Could you check a few things on this model? Use its own coordinates, in mm. A direction names the side the tool comes from. Give positions to 0.01 mm unless a question says otherwise; leave off trailing zeros. Order: outer loops, then holes, each group sorted by start corner. A loop starts at its lowest first (then second) coordinate and runs counter-clockwise, first axis right, second up.
from build123d import *

# Parameters (mm, degrees)
F1_DEPTH = 5
F3_DEPTH = 3
F4_DEPTH = 16


with BuildPart() as f1:
    # F0 (on Front) → F1 (new body, symmetric)
    with BuildSketch(Plane.XZ):
        with BuildLine():
            ThreePointArc((0, -4), (-4, 0), (0, 4))
            Line((0, 4), (0, 8))
            ThreePointArc((0, 8), (-6.9282032303, 4), (-6.9282032303, -4))
            Line((-6.9282032303, -4), (0, -4))
        make_face()
        with BuildLine():
            Line((31.6095426679, 8), (0, 8))
            ThreePointArc((0, 8), (4, 6.9282032303), (6.9282032303, 4))
            Line((6.9282032303, 4), (31.6095426679, 4))
            Line((31.6095426679, 4), (31.6095426679, 8))
        make_face()
        with BuildLine():
            Line((0, 8), (0, 4))
            Line((0, 4), (2.413712136, 4))
            Line((2.413712136, 4), (6.9282032303, 4))
            ThreePointArc((6.9282032303, 4), (4, 6.9282032303), (0, 8))
        make_face()
        with BuildLine():
            Line((31.6095426679, -4), (6.9282032303, -4))
            ThreePointArc((6.9282032303, -4), (4.4598401279, -6.6415228701), (1.0806620306, -7.9266745597))
            Line((1.0806620306, -7.9266745597), (31.6095426679, -7.9266745597))
            Line((31.6095426679, -7.9266745597), (31.6095426679, -4))
        make_face()
        with BuildLine():
            ThreePointArc((-1.0806620306, -7.9266745597), (-4.4598401279, -6.6415228701), (-6.9282032303, -4))
            Line((-6.9282032303, -4), (-40.4233634472, -4))
            Line((-40.4233634472, -4), (-40.4233634472, -7.9266745597))
            Line((-40.4233634472, -7.9266745597), (-1.0806620306, -7.9266745597))
        make_face()
        with BuildLine():
            Line((0, -7.9266745597), (0, -4))
            Line((0, -4), (-6.9282032303, -4))
            ThreePointArc((-6.9282032303, -4), (-4.4598401279, -6.6415228701), (-1.0806620306, -7.9266745597))
            Line((-1.0806620306, -7.9266745597), (0, -7.9266745597))
        make_face()
        with BuildLine():
            Line((2.413712136, -4), (0, -4))
            Line((0, -4), (0, -7.9266745597))
            Line((0, -7.9266745597), (1.0806620306, -7.9266745597))
            ThreePointArc((1.0806620306, -7.9266745597), (4.4598401279, -6.6415228701), (6.9282032303, -4))
            Line((6.9282032303, -4), (2.413712136, -4))
        make_face()
        with BuildLine():
            Line((2.413712136, 4), (2.413712136, 3.1896698457))
            Line((2.413712136, 3.1896698457), (7.3366209031, 3.1896698457))
            ThreePointArc((7.3366209031, 3.1896698457), (7.1439107377, 3.6006304131), (6.9282032303, 4))
            Line((6.9282032303, 4), (2.413712136, 4))
        make_face()
        with BuildLine():
            ThreePointArc((6.9282032303, 4), (7.1439107377, 3.6006304131), (7.3366209031, 3.1896698457))
            Line((7.3366209031, 3.1896698457), (31.6095426679, 3.1896698457))
            Line((31.6095426679, 3.1896698457), (31.6095426679, 4))
            Line((31.6095426679, 4), (6.9282032303, 4))
        make_face()
        with BuildLine():
            Line((7.3366209031, -3.1896698457), (2.413712136, -3.1896698457))
            Line((2.413712136, -3.1896698457), (2.413712136, -4))
            Line((2.413712136, -4), (6.9282032303, -4))
            ThreePointArc((6.9282032303, -4), (7.1439107377, -3.6006304131), (7.3366209031, -3.1896698457))
        make_face()
        with BuildLine():
            Line((2.413712136, -4), (2.413712136, -3.1896698457))
            ThreePointArc((2.413712136, -3.1896698457), (1.2730515734, -3.7920099804), (0, -4))
            Line((0, -4), (2.413712136, -4))
        make_face()
        with BuildLine():
            ThreePointArc((0, 4), (1.2730515734, 3.7920099804), (2.413712136, 3.1896698457))
            Line((2.413712136, 3.1896698457), (2.413712136, 4))
            Line((2.413712136, 4), (0, 4))
        make_face()
        with BuildLine():
            Line((31.6095426679, -3.1896698457), (7.3366209031, -3.1896698457))
            ThreePointArc((7.3366209031, -3.1896698457), (7.1439107377, -3.6006304131), (6.9282032303, -4))
            Line((6.9282032303, -4), (31.6095426679, -4))
            Line((31.6095426679, -4), (31.6095426679, -3.1896698457))
        make_face()
    extrude(amount=F1_DEPTH, both=True)

    # F2 (on face) → F3 (join)
    with BuildSketch(Plane.XY.offset(8)):
        Polygon((26.3679362833, -2.1467979489), (26.3679362833, 2.1467979489), (22.6495731622, 4.2935958979), (18.931210041, 2.1467979489), (18.931210041, -2.1467979489), (22.6495731622, -4.2935958979), align=None)
        Polygon((23.6495732055, 1.7320507826), (24.6495731622, 1.1547005384), (24.6495731622, 0), (24.6495731622, -1.1547005384), (23.6495731174, -1.7320508334), (22.6495731622, -2.3094010768), (21.6495731189, -1.7320507826), (20.6495731622, -1.1547005384), (20.6495731622, 0), (20.6495731622, 1.1547005384), (21.6495731525, 1.732050802), (22.6495731622, 2.3094010768), align=None, mode=Mode.SUBTRACT)
    extrude(amount=F3_DEPTH)

    # F2 (on face) → F4 (cut)
    with BuildSketch(Plane.XY.offset(8)):
        with BuildLine():
            ThreePointArc((23.6495731174, -1.7320508334), (24.3816239568, -1.0000000224), (24.6495731622, 0))
            ThreePointArc((24.6495731622, 0), (24.3816239823, 0.9999999783), (23.6495732055, 1.7320507826))
            ThreePointArc((23.6495732055, 1.7320507826), (22.6495731816, 2), (21.6495731525, 1.732050802))
            ThreePointArc((21.6495731525, 1.732050802), (20.9175223518, 0.9999999952), (20.6495731622, 0))
            ThreePointArc((20.6495731622, 0), (20.9175223421, -0.9999999783), (21.6495731189, -1.7320507826))
            ThreePointArc((21.6495731189, -1.7320507826), (22.6495731113, -2), (23.6495731174, -1.7320508334))
        make_face()
    extrude(amount=-F4_DEPTH, mode=Mode.SUBTRACT)


solid = f1.part
Item 1: Imagine slicing it at B-B on z = 6. List the corners of the cut face in (x, y) for me.
Findings:
outline: (-5.29, -5) - (31.61, -5) - (31.61, 5) - (-5.29, 5) - close; hole circle Ø4 at (22.65, 0)
Item 2: Imagine slicing it at A-A on x = 16.5. List the corners of the cut face in (y, z) for me, then the cut area to 3 significant figures.
Findings:
outline: (-5, -7.93) - (5, -7.93) - (5, -3.19) - (-5, -3.19) - close; (-5, 3.19) - (5, 3.19) - (5, 8) - (-5, 8) - close
area: 95.5 mm2
Item 3: Imagine slicing it at C-C on y = -3.25. List the corners of the cut face in (x, z) for me.
Findings:
outline: (-40.42, -7.93) - (31.61, -7.93) - (31.61, -3.19) - (2.41, -3.19) arc R4 cw (long way) to (2.41, 3.19) - (31.61, 3.19) - (31.61, 8) - (24.46, 8) - (24.46, 11) - (20.84, 11) - (20.84, 8) - (0, 8) arc R8 ccw to (-6.93, -4) - (-40.42, -4) - close
Item 4: For faces 4 (the flat face through (20.816, 3.235, 9.479)), 5 (the flat face through (18.931, 0, 9)), 6 (the flat face through (24.53, 3.21, 9.48)), which set-ups out of +Z, -Z, +X, -X, +Y, -Y let a thin tool reach every point of the face, with its end or its side?
Findings:
face 4: +Z, -X, +Y
face 5: +Z, -X, +Y, -Y
face 6: +Z, +X, +Y
Item 5: Please list where these lines run through material, in increasing order: line 1 along Z through (x, y) = (17, -1.25); line 2 along Z through (x, y) = (-13.5, -2); line 3 along Z through (x, y) = (-1, 1.75).
Findings:
line 1: z = -7.93 to -3.19, 3.19 to 8
line 2: z = -7.93 to -4
line 3: z = -7.93 to -3.87, 3.87 to 7.94
Item 6: We'd pull the mould along Z, two halves only. Please class faces 1 (the flat face through (17, 0, -3.19)), 2 (the flat face through (24.483, -3.235, 9.479)), 3 (the flat face through (21, -2, 11)): +Z half, -Z half, draft (parallel to the pull), parting line (faces both ways), or undercut.
Findings:
face 1: undercut
face 2: draft
face 3: +Z half
Item 7: Imagine slicing it at D-D on z = 0. List the corners of the cut face in (x, y) for me.
Findings:
outline: (-8, -5) - (-4, -5) - (-4, 5) - (-8, 5) - close
Item 8: For pin 1 (1.8 mm diameter, centred on y = 0, z = 10, fed in from -X); pin 2 (6 mm diameter, centred on x = -17.5, y = -3, fed in from +Z); pin 3 (6 mm diameter, centred on y = -4, z = 1.5, fed in from -X), each with a flat end and sliding along its axis, tell me the tip position at first contact or that it passes through.
Findings:
pin 1: stops at x = 18.93
pin 2: stops at z = -4
pin 3: stops at x = -8
